```python
from build123d import *

# Parameters (mm, degrees)
SKETCH_1_W          = 14
SKETCH_1_H          = 2.5
SKETCH_1_R          = 1.7
SKETCH_1_R_2        = 11.75
SKETCH_1_R_3        = 2.2
SKETCH_1_W_2        = 4.5
SKETCH_1_H_2        = 20
EXTRUDE_1_DEPTH     = 5
EXTRUDE_2_DEPTH     = 60
CUT_EXTRUDE_1_REACH = 78.223
CUT_EXTRUDE_2_REACH = 78.223
SKETCH_2_3_R        = 1
EXTRUDE_3_DEPTH     = 5
FILLET_1_R          = 5
FILLET_START        = 22.5
FILLET_2_DEPTH      = 5
FILLET_START_2      = -60
FILLET_2_2_DEPTH    = 61.119099979
FILLET_START_3      = 27.5
FILLET_2_3_DEPTH    = 3
FILLET_3_R          = 2


with BuildPart() as part:
    # 草图1 → 凸台-拉伸1 (new body)
    # profile 1 of 9: a face of its own
    with BuildSketch(Plane.XY):
        with Locations((34, 21.75)):
            Rectangle(SKETCH_1_W, SKETCH_1_H)
    # profile 2 of 9: a face of its own
    with BuildSketch(Plane.XY):
        Polygon((27, 23), (22.5, 23), (22.5, 21.5), (22.5, 10), (27, 10), (27, 20.5), align=None)
    # profile 3 of 9: a face of its own
    with BuildSketch(Plane.XY):
        Polygon((-21, 23), (-21, 21.5), (21, 21.5), (22.5, 21.5), (22.5, 23), align=None)
    # profile 4 of 9: a face of its own
    with BuildSketch(Plane.XY):
        Polygon((21, 21.5), (-21, 21.5), (-21, -21.5), (21, -21.5), (22.5, -21.5), (22.5, -10), (22.5, 10), (22.5, 21.5), align=None)
        with Locations((-15.68126777, -15.316587124)):
            Circle(SKETCH_1_R, mode=Mode.SUBTRACT)
        with Locations((15.316587124, -15.68126777)):
            Circle(SKETCH_1_R, mode=Mode.SUBTRACT)
        Circle(SKETCH_1_R_2, mode=Mode.SUBTRACT)
        with Locations((-15.316587124, 15.68126777)):
            Circle(SKETCH_1_R, mode=Mode.SUBTRACT)
        with Locations((15.68126777, 15.316587124)):
            Circle(SKETCH_1_R, mode=Mode.SUBTRACT)
    # profile 5 of 9: a face of its own
    with BuildSketch(Plane.XY):
        Polygon((41, 20.5), (27, 20.5), (27, 10), (27, -10), (27, -20.5), (41, -20.5), align=None)
        with Locations((33, -10)):
            Circle(SKETCH_1_R_3, mode=Mode.SUBTRACT)
        with Locations((33, 10)):
            Circle(SKETCH_1_R_3, mode=Mode.SUBTRACT)
    # profile 6 of 9: a face of its own
    with BuildSketch(Plane.XY):
        with Locations((24.75, 0)):
            Rectangle(SKETCH_1_W_2, SKETCH_1_H_2)
    # profile 7 of 9: a face of its own
    with BuildSketch(Plane.XY):
        Polygon((22.5, -10), (22.5, -21.5), (22.5, -23), (27, -23), (27, -20.5), (27, -10), align=None)
    # profile 8 of 9: a face of its own
    with BuildSketch(Plane.XY):
        with Locations((34, -21.75)):
            Rectangle(SKETCH_1_W, SKETCH_1_H)
    # profile 9 of 9: a face of its own
    with BuildSketch(Plane.XY):
        Polygon((21, -21.5), (-21, -21.5), (-21, -23), (22.5, -23), (22.5, -21.5), align=None)
    extrude(amount=EXTRUDE_1_DEPTH)

    # 草图1<4> → 凸台-拉伸2 (add)
    with BuildSketch(Plane.XY):
        Polygon((22.5, 23), (22.5, 10), (27, 10), (27, 20.5), (41, 20.5), (41, 23), align=None)
        Polygon((22.5, -10), (22.5, -23), (41, -23), (41, -20.5), (27, -20.5), (27, -10), align=None)
    extrude(amount=-EXTRUDE_2_DEPTH)

    # 草图2 → 切除-拉伸1 (cut, up to next)
    with BuildSketch(Plane(origin=(0, 0, 0), x_dir=(1, 0, 0), z_dir=(0, 1, 0)), mode=Mode.PRIVATE) as cut_extrude_1_sk1:
        with BuildLine():
            ThreePointArc((37.7, 10), (35.5, 12.2), (33.3, 10))
            Line((33.3, 10), (37.7, 10))
        make_face()
    cut_extrude_1_tool1 = extrude(cut_extrude_1_sk1.sketch, amount=-CUT_EXTRUDE_1_REACH, mode=Mode.PRIVATE) & part.part
    # 草图2 → 切除-拉伸1 (cut, up to next)
    with BuildSketch(Plane(origin=(0, 0, 0), x_dir=(1, 0, 0), z_dir=(0, 1, 0)), mode=Mode.PRIVATE) as cut_extrude_1_sk2:
        with BuildLine():
            Line((37.7, 10), (33.3, 10))
            ThreePointArc((33.3, 10), (35.5, 7.8), (37.7, 10))
        make_face()
    cut_extrude_1_tool2 = extrude(cut_extrude_1_sk2.sketch, amount=-CUT_EXTRUDE_1_REACH, mode=Mode.PRIVATE) & part.part
    # 草图2 → 切除-拉伸1 (cut, up to next)
    with BuildSketch(Plane(origin=(0, 0, 0), x_dir=(1, 0, 0), z_dir=(0, 1, 0)), mode=Mode.PRIVATE) as cut_extrude_1_sk3:
        with BuildLine():
            ThreePointArc((37.7, 10), (35.5, 12.2), (33.3, 10))
            Line((33.3, 10), (37.7, 10))
        make_face()
    cut_extrude_1_tool3 = extrude(cut_extrude_1_sk3.sketch, amount=-CUT_EXTRUDE_1_REACH, mode=Mode.PRIVATE) & part.part
    # 草图2 → 切除-拉伸1 (cut, up to next)
    with BuildSketch(Plane(origin=(0, 0, 0), x_dir=(1, 0, 0), z_dir=(0, 1, 0)), mode=Mode.PRIVATE) as cut_extrude_1_sk4:
        with BuildLine():
            Line((37.7, 10), (33.3, 10))
            ThreePointArc((33.3, 10), (35.5, 7.8), (37.7, 10))
        make_face()
    cut_extrude_1_tool4 = extrude(cut_extrude_1_sk4.sketch, amount=-CUT_EXTRUDE_1_REACH, mode=Mode.PRIVATE) & part.part
    add(cut_extrude_1_tool1.solids().sort_by_distance((35.5, 0, -10.933709))[0], mode=Mode.SUBTRACT)
    add(cut_extrude_1_tool2.solids().sort_by_distance((35.5, 0, -9.066291))[0], mode=Mode.SUBTRACT)
    add(cut_extrude_1_tool3.solids().sort_by_distance((35.5, 0, -10.933709))[0], mode=Mode.SUBTRACT)
    add(cut_extrude_1_tool4.solids().sort_by_distance((35.5, 0, -9.066291))[0], mode=Mode.SUBTRACT)

    # 草图2<3> → 切除-拉伸2 (cut, up to next)
    with BuildSketch(Plane(origin=(0, 0, 0), x_dir=(1, 0, 0), z_dir=(0, 1, 0)), mode=Mode.PRIVATE) as cut_extrude_2_sk1:
        with Locations(Location((37, 7, 0), (0, 0, 90))):
            Circle(SKETCH_2_3_R)
    cut_extrude_2_tool1 = extrude(cut_extrude_2_sk1.sketch, amount=CUT_EXTRUDE_2_REACH, mode=Mode.PRIVATE) & part.part
    # 草图2<3> → 切除-拉伸2 (cut, up to next)
    with BuildSketch(Plane(origin=(0, 0, 0), x_dir=(1, 0, 0), z_dir=(0, 1, 0)), mode=Mode.PRIVATE) as cut_extrude_2_sk2:
        with Locations(Location((37, 13, 0), (0, 0, 90))):
            Circle(SKETCH_2_3_R)
    cut_extrude_2_tool2 = extrude(cut_extrude_2_sk2.sketch, amount=CUT_EXTRUDE_2_REACH, mode=Mode.PRIVATE) & part.part
    add(cut_extrude_2_tool1.solids().sort_by_distance((37, 0, -7))[0], mode=Mode.SUBTRACT)
    add(cut_extrude_2_tool2.solids().sort_by_distance((37, 0, -13))[0], mode=Mode.SUBTRACT)

    # 草图5 → 凸台-拉伸3 (add)
    with BuildSketch(Plane.ZY.offset(-22.5)):
        Polygon((-60, 75), (-60, 23), (0, 23), align=None)
        Polygon((0, -23), (-60, -23), (-60, -75), align=None)
    extrude(amount=-EXTRUDE_3_DEPTH)

    # 圆角1
    fillet_1_edges = [part.edges().sort_by_distance(p)[0] for p in [
        (25, -75, -60),
        (25, 75, -60),
        (-21, -23, 2.5),
        (-21, 23, 2.5),
    ]]
    fillet(fillet_1_edges, radius=FILLET_1_R)

    # 圆角2: read off the stored shape, not the designer's step
    # 圆角2 outline → 圆角2 (add)
    with BuildSketch(Plane.YZ.offset(FILLET_START)):
        with BuildLine():
            ThreePointArc((-23, 1.119099979), (-23.189199247, 0.070577625), (-23.732932752, -0.845691636))
            Line((-23.732932752, -0.845691636), (-23, 0))
            Line((-23, 0), (-23, 1.119099979))
        make_face()
        with BuildLine():
            Line((23, 0), (23.732932752, -0.845691636))
            ThreePointArc((23.732932752, -0.845691636), (23.189199247, 0.070577625), (23, 1.119099979))
            Line((23, 1.119099979), (23, 0))
        make_face()
    extrude(amount=FILLET_2_DEPTH)

    # Fillet 2 2 outline → Fillet 2 2 (add)
    with BuildSketch(Plane.XY.offset(FILLET_START_2)):
        with BuildLine():
            Line((27.5, -23), (27.5, -26))
            ThreePointArc((27.5, -26), (28.378679656, -23.878679656), (30.5, -23))
            Line((30.5, -23), (27.5, -23))
        make_face()
        with BuildLine():
            Line((27.5, 23), (30.5, 23))
            ThreePointArc((30.5, 23), (28.378679656, 23.878679656), (27.5, 26))
            Line((27.5, 26), (27.5, 23))
        make_face()
    extrude(amount=FILLET_2_2_DEPTH)

    # Fillet 2 3 outline → Fillet 2 3 (cut)
    with BuildSketch(Plane.YZ.offset(FILLET_START_3)):
        with BuildLine():
            Line((-27.333333343, -5), (-23.732932752, -0.845691636))
            ThreePointArc((-23.732932752, -0.845691636), (-23.189199247, 0.070577625), (-23, 1.119099979))
            Line((-23, 1.119099979), (-28, 1.119099979))
            Line((-28, 1.119099979), (-28, -5))
            Line((-28, -5), (-27.333333343, -5))
        make_face()
        with BuildLine():
            Line((23.732932752, -0.845691636), (27.333333343, -5))
            Line((27.333333343, -5), (28, -5))
            Line((28, -5), (28, 1.119099979))
            Line((28, 1.119099979), (23, 1.119099979))
            ThreePointArc((23, 1.119099979), (23.189199247, 0.070577625), (23.732932752, -0.845691636))
        make_face()
    extrude(amount=FILLET_2_3_DEPTH, mode=Mode.SUBTRACT)

    # 圆角3
    fillet_3_edges = [part.edges().sort_by_distance(p)[0] for p in [
        (-21, 0, 5),
        (12.5, 23, 5),
        (-19.535533906, 21.535533906, 5),
        (-19.535533906, -21.535533906, 5),
        (12.5, -23, 5),
    ]]
    fillet(fillet_3_edges, radius=FILLET_3_R)


solid = part.part
```
The model under review builds one solid part; all positions refer to its coordinate system, in mm. A direction names the side the tool comes from. Round coordinates to 2 decimals unless told otherwise and drop trailing zeros. Loops run counter-clockwise (first coordinate to the right, second up) from the corner with the lowest first, then second, coordinate; pieces in that order, holes last.
1) Consider section D-D on z = -10. State the section outline as (x, y) points.
Values follow:
outline: (22.5, -31.67) - (27.5, -31.67) - (27.5, -26) arc R3 cw to (30.5, -23) - (33.3, -23) - (33.3, -20.5) - (27, -20.5) - (27, -10) - (22.5, -10) - close; (22.5, 10) - (27, 10) - (27, 20.5) - (41, 20.5) - (41, 23) - (30.5, 23) arc R3 cw to (27.5, 26) - (27.5, 31.67) - (22.5, 31.67) - close; (37.7, -23) - (41, -23) - (41, -20.5) - (37.7, -20.5) - close
2) Consider section C-C on z = -40. State the section outline as (x, y) points, then the cut area to 3 significant figures.
Values follow:
outline: (22.5, -57.67) - (27.5, -57.67) - (27.5, -26) arc R3 cw to (30.5, -23) - (41, -23) - (41, -20.5) - (27, -20.5) - (27, -10) - (22.5, -10) - close; (22.5, 10) - (27, 10) - (27, 20.5) - (41, 20.5) - (41, 23) - (30.5, 23) arc R3 cw to (27.5, 26) - (27.5, 57.67) - (22.5, 57.67) - close
area: 538 mm2
3) The part is to be moulded in two halves that separate along Y. For faces 1 (the face through (25, -10, -30)), 2 (the face through (31, -23, -26)), 3 (the face through (26, 35, -60)), 4 (the face through (27, -15, -30)), say which applies: pulls with the +Y half, pulls with the -Y half, needs draft (parallel to the pull), parting line crosses it, or undercut.
Values follow:
face 1: undercut
face 2: pulls with the -Y half
face 3: needs draft
face 4: undercut
4) Consider section B-B on x = 1. State the section outline as (y, z) points, then the cut area to 3 significant figures.
Values follow:
outline: (-23, 0) - (-11.71, 0) - (-11.71, 5) - (-21, 5) arc R2 ccw to (-23, 3) - close; (11.71, 0) - (23, 0) - (23, 3) arc R2 ccw to (21, 5) - (11.71, 5) - close
area: 111 mm2
5) Tool access review of faces 5 (the face through (27, 15, -30)), 6 (the face through (30.802, 10.097, 2.465)), 7 (the face through (25, 10, -30)), 8 (the face through (27.5, -43, -38)), 9 (the face through (26, -35, -60)): name each direction out of +Z, -Z, +X, -X, +Y, -Y from which nothing blocks a thin tool from reaching the whole face with its end or side.
Values follow:
face 5: -Z, +X
face 6: +Z, -Z
face 7: -Z, +X, -X
face 8: +Z, -Z, +X, -Y
face 9: -Z, +X, -X, +Y, -Y
6) Wall thickness on line 1 along Y through (x, z) = (33, 2.05); line 2 along X through (y, z) = (29, -8); line 3 along X through (y, z) = (-15.5, -33.5): over which ranges is each line inside the solid? List them lowest first.
Values follow:
line 1: y = -23 to -12.2, -7.8 to 7.8, 12.2 to 23
line 2: x = 22.5 to 27.5
line 3: x = 22.5 to 27
7) Clearance check with flat-ended pins moving along their axes: P1, Ø3, axis at y = 13.5, z = -31.5, coming from the +X side; P2, Ø2.5, axis at x = 35.5, z = -10, coming from the +Y side; P3, Ø12, axis at x = 13, y = -34, coming from the -Z side; P4, Ø5, axis at x = 15, y = -23, coming from the -Z side. State where each tip first meets the part, or that it passes through.
Values follow:
P1: stops at x = 27
P2: stops at y = 23
P3: passes through
P4: stops at z = 0
8) Consider section A-A on y = 0. State the section outline as (x, z) points.
Values follow:
outline: (-21, 0) - (-11.75, 0) - (-11.75, 5) - (-19, 5) arc R2 ccw to (-21, 3) - close; (11.75, 0) - (41, 0) - (41, 5) - (11.75, 5) - close
